Could you check a few things on this model? Use its own coordinates, in mm. Give positions to 0.01 mm unless a question says otherwise; leave off trailing zeros.
(1) If we mould it in two halves opening along Y, with no side actions, what happens to faces 1 (the flat face through (-19, 5, 20)), 2 (the flat face through (-5.205, 14.471, 0.684)), 3 (the flat face through (-15, 5, 18))? For each: released by +Y, released by -Y, zero draft, split by the parting line, or undercut.
(2) If I drill on probe 1 along Z at (x, y) = (-11.5, 5), over which ranges is the centre line in solid material (lowest first)?
(3) Will these pins go through, and if not, where does the flat tip stop? pin 1 (0.9 mm diameter, centred on x = -14, y = 5, fed in from +Z); pin 2 (8 mm diameter, centred on x = -17, y = 5.5, fed in from +Z).
from build123d import *

# Parameters (mm, degrees)
SKETCH_2_W          = 20
SKETCH_2_H          = 20
EXTRUDE_1_DEPTH     = 20
CHAMFER_2_SIZE      = 1
SKETCH_3_R          = 3.5
CUT_EXTRUDE_1_DEPTH = 2
FILLET_1_R          = 2


with BuildPart() as part:
    # ｽｹｯﾁ2 → ﾎﾞｽ - 押し出し1 (new body)
    with BuildSketch(Plane.XY):
        with Locations((-14.586466165, 5.169172932)):
            Rectangle(SKETCH_2_W, SKETCH_2_H)
    extrude(amount=EXTRUDE_1_DEPTH)

    # 面取り2
    chamfer_2_edges = [part.edges().sort_by_distance(p)[0] for p in [
        (-4.586466165, 5.169172932, 20),
        (-14.586466165, 15.169172932, 20),
        (-24.586466165, 5.169172932, 20),
        (-14.586466165, 15.169172932, 0),
        (-4.586466165, 5.169172932, 0),
        (-24.586466165, 15.169172932, 10),
        (-4.586466165, 15.169172932, 10),
        (-4.586466165, -4.830827068, 10),
        (-14.586466165, -4.830827068, 20),
    ]]
    chamfer(chamfer_2_edges, length=CHAMFER_2_SIZE)

    # ｽｹｯﾁ3 → ｶｯﾄ - 押し出し1 (cut)
    with BuildSketch(Plane.XY.offset(20)):
        with Locations((-14.586466165, 5.169172932)):
            Circle(SKETCH_3_R)
    extrude(amount=-CUT_EXTRUDE_1_DEPTH, mode=Mode.SUBTRACT)

    # ﾌｨﾚｯﾄ1
    fillet_1_edges = [part.edges().sort_by_distance(p)[0] for p in [
        (-18.086466165, 5.169172932, 18),
    ]]
    fillet(fillet_1_edges, radius=FILLET_1_R - 0.0001)  # a hair under: the kernel refuses the full size


solid = part.part
Answer block:
1. face 1: zero draft
1. face 2: released by +Y
1. face 3: undercut
2. probe 1: z = 0 to 18.79
3. pin 1: stops at z = 18
3. pin 2: stops at z = 20
